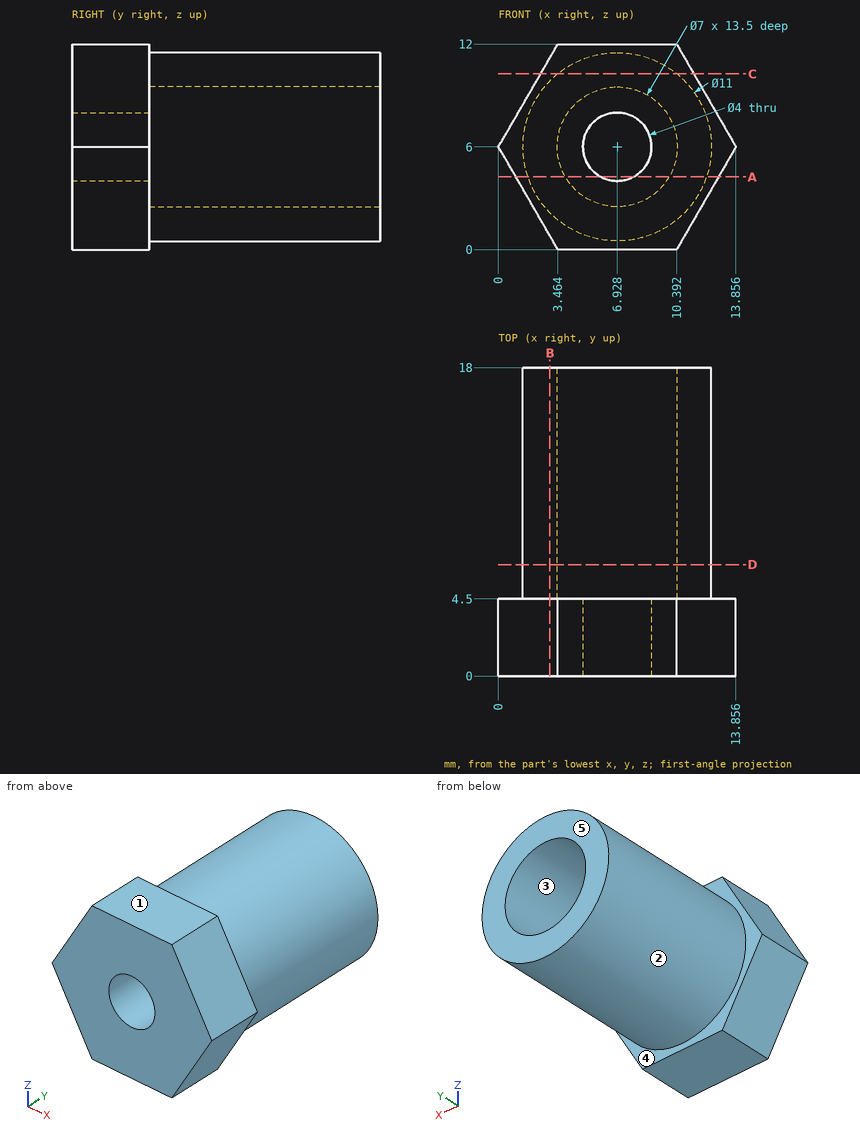
Print and shaded views of the part. All mm, measured from the part's lowest x, y and z. A direction names the side the tool comes from. Give positions to 0.01 mm unless a question says otherwise; leave off trailing zeros. Loops run counter-clockwise (first coordinate to the right, second up) from the corner with the lowest first, then second, coordinate; pieces in that order, holes last. Notation, with made-up numbers: (53, -38) -> (78, -38) arc R12 ccw to (78, -15) -> close; hole circle Ø9 at (37, -5.5). An arc over 180 degrees is marked (long way). Use CSV: the item, a comma, the result in double quotes. Start each with the question number.
1) Slice it at B-B on x = 3. Give the cut face in (y, z), plus the area to 3 significant figures.
2) Slice it at C-C on z = 10.25. Give the cut face in (x, y).
3) Wall check: line 1 (Y direction, x = 9, z = 6.75); line 2 (X direction, y = 9.5, z = 6); line 3 (Z direction, x = 6, y = 2.25). Give the ranges that are in metal, low to high.
4) Tool access for the marked faces 4 and 5: list every direction of +Z, -Z, +X, -X, +Y, -Y with a clear straight run to the whole face (end or side of a thin tool).
5) Mould opens along Z. For the marked faces 1, 2 and 3 say: released by +Z, released by -Z, zero draft, split by the parting line, or undercut.
6) Flat gauge pins, fed straight in: pin 1 Ø3 at (y, z) = (4, 8) entering from +X; pin 2 Ø4 at (x, y) = (11.5, 9) entering from -Z; pin 3 Ø1 at (y, z) = (14, 9) entering from -X. Where does each tip first touch, or does it go through?
7) Slice it at A-A on z = 4.25. Give the cut face in (x, y).
8) Slice it at D-D on y = 6.5. Give the cut face in (x, z).
Computed values:
1,outline,"(0, 0.8) -> (4.5, 0.8) -> (4.5, 2.15) -> (18, 2.15) -> (18, 9.85) -> (4.5, 9.85) -> (4.5, 11.2) -> (0, 11.2) -> close"
1,area,"151 mm^2"
2,outline,"(2.45, 0) -> (11.4, 0) -> (11.4, 4.5) -> (10.42, 4.5) -> (10.42, 18) -> (3.44, 18) -> (3.44, 4.5) -> (2.45, 4.5) -> close"
3,line 1,"y = 0 to 4.5"
3,line 2,"x = 1.43 to 3.43, 10.43 to 12.43"
3,line 3,"z = 0 to 4.23, 7.77 to 12"
4,face 4,"+Y"
4,face 5,"+Z, -Z, +X, -X, +Y"
5,face 1,"released by +Z"
5,face 2,"split by the parting line"
5,face 3,"undercut"
6,pin 1,"stops at x = 13.57"
6,pin 2,"stops at z = 1.14"
6,pin 3,"stops at x = 2.03"
7,outline,"(1.01, 0) -> (5.96, 0) -> (5.96, 4.5) -> (3.9, 4.5) -> (3.9, 18) -> (1.71, 18) -> (1.71, 4.5) -> (1.01, 4.5) -> close; (7.9, 0) -> (12.85, 0) -> (12.85, 4.5) -> (12.14, 4.5) -> (12.14, 18) -> (9.96, 18) -> (9.96, 4.5) -> (7.9, 4.5) -> close"
8,outline,"circle Ø11 at (6.93, 6); hole circle Ø7 at (6.93, 6)"
